Geometry: final body of the model. Coordinates: model frame, mm. Give positions to 0.01 mm unless a question says otherwise; leave off trailing zeros. Loops run counter-clockwise (first coordinate to the right, second up) from the corner with the lowest first, then second, coordinate; pieces in that order, holes last. Notation, with made-up numbers: (44.25, 73) - (49.25, 73) arc R17 ccw to (49.25, 83) - close; hole circle Ø11 at (83.5, 42.5). An arc over 180 degrees is marked (long way). Answer in a Markdown table with one row per item.
from build123d import *

# Parameters (mm, degrees)
F0_W           = 48
F0_H           = 48
F1_DEPTH       = 48
F2_R           = 1
F3_R           = 1
F4_T1_DEPTH    = 46
F4_T3_DEPTH    = 46
F4_T5_DEPTH    = 46
F4_S9_W        = 1
F4_S9_H        = 1
F4_T10_DEPTH   = 1
F4_S15_W       = 1
F4_S15_H       = 1
F4_T16_DEPTH   = 1
F4_S21_W       = 1
F4_S21_H       = 1
F4_T22_DEPTH   = 1
F4_S27_W       = 1
F4_S27_H       = 1
F4_T28_DEPTH   = 1
F4_T32_ANGLE   = 90
F4_T34_ANGLE   = 90
F6_D           = 18
F6_CSINK_D     = 36
F6_CSINK_ANGLE = 45


# Not quite as in the source:
# - a fillet or chamfer that OpenCascade refuses, or shapes differently, is made with other operations: its cross-section is extruded or revolved along the edge and cut away or added


with BuildPart() as f1:
    # F0 (on Front) → F1 (new body)
    with BuildSketch(Plane.XZ):
        Rectangle(F0_W, F0_H)
    extrude(amount=F1_DEPTH)

    # F2
    f2_edges = [f1.edges().sort_by_distance(p)[0] for p in [
        (24, -24, 24),
    ]]
    fillet(f2_edges, radius=F2_R)

    # F3
    f3_edges = [f1.edges().sort_by_distance(p)[0] for p in [
        (-24, -24, 24),
        (-0.5, 0, 24),
        (-0.5, -48, 24),
    ]]
    fillet(f3_edges, radius=F3_R)

    # F4: fillet of radius 1 on 8 edges, made by hand

    # F4_s2 → F4_t1 (cut)
    with BuildSketch(Plane.XY.offset(-23)):
        with BuildLine():
            ThreePointArc((-23, -48), (-23.7071067812, -47.7071067812), (-24, -47))
            Line((-24, -47), (-24, -48))
            Line((-24, -48), (-23, -48))
        make_face()
        with BuildLine():
            ThreePointArc((-23, 0), (-23.7071067812, -0.2928932188), (-24, -1))
            Line((-24, -1), (-24, 0))
            Line((-24, 0), (-23, 0))
        make_face()
    extrude(amount=F4_T1_DEPTH, mode=Mode.SUBTRACT)

    # F4_s4 → F4_t3 (cut)
    with BuildSketch(Plane.YZ.offset(-23)):
        with BuildLine():
            ThreePointArc((0, -23), (-0.2928932188, -23.7071067812), (-1, -24))
            Line((-1, -24), (0, -24))
            Line((0, -24), (0, -23))
        make_face()
        with BuildLine():
            ThreePointArc((-48, -23), (-47.7071067812, -23.7071067812), (-47, -24))
            Line((-47, -24), (-48, -24))
            Line((-48, -24), (-48, -23))
        make_face()
    extrude(amount=F4_T3_DEPTH, mode=Mode.SUBTRACT)

    # F4_s6 → F4_t5 (cut)
    with BuildSketch(Plane.XZ.offset(1)):
        with BuildLine():
            ThreePointArc((-24, -23), (-23.7071067812, -23.7071067812), (-23, -24))
            Line((-23, -24), (-24, -24))
            Line((-24, -24), (-24, -23))
        make_face()
        with BuildLine():
            ThreePointArc((24, -23), (23.7071067812, -23.7071067812), (23, -24))
            Line((23, -24), (24, -24))
            Line((24, -24), (24, -23))
        make_face()
    extrude(amount=F4_T5_DEPTH, mode=Mode.SUBTRACT)


with BuildPart() as f4_tool8:
    # F4_s9 → F4_t10 (new body)
    with BuildSketch(Plane.XZ.offset(1)):
        with Locations((-23.5, 23.5)):
            Rectangle(F4_S9_W, F4_S9_H)
    extrude(amount=-F4_T10_DEPTH)

    # F4_s11 → F4_t12 (revolve, cut)
    with BuildSketch(Plane(origin=(-23, -1, 23), x_dir=(0.7071067812, 0, -0.7071067812), z_dir=(0.7071067812, 0, 0.7071067812))):
        with BuildLine():
            ThreePointArc((0, -1), (1, 0), (0, 1))
            Line((0, 1), (0, -1))
        make_face()
    revolve(axis=Axis((-23, -1, 23), (0, 1, 0)), mode=Mode.SUBTRACT)


with BuildPart() as f1_1:
    add(f1.part)

    # F4_t7: cut F4_tool8
    add(f4_tool8.part, mode=Mode.SUBTRACT)


with BuildPart() as f4_tool14:
    # F4_s15 → F4_t16 (new body)
    with BuildSketch(Plane.XZ.offset(47)):
        with Locations((-23.5, 23.5)):
            Rectangle(F4_S15_W, F4_S15_H)
    extrude(amount=F4_T16_DEPTH)

    # F4_s17 → F4_t18 (revolve, cut)
    with BuildSketch(Plane(origin=(-23, -47, 23), x_dir=(0.7071067812, 0, -0.7071067812), z_dir=(-0.7071067812, 0, -0.7071067812))):
        with BuildLine():
            ThreePointArc((0, -1), (1, 0), (0, 1))
            Line((0, 1), (0, -1))
        make_face()
    revolve(axis=Axis((-23, -47, 23), (0, -1, 0)), mode=Mode.SUBTRACT)


with BuildPart() as f1_2:
    add(f1_1.part)

    # F4_t13: cut F4_tool14
    add(f4_tool14.part, mode=Mode.SUBTRACT)


with BuildPart() as f4_tool20:
    # F4_s21 → F4_t22 (new body)
    with BuildSketch(Plane.XZ.offset(47)):
        with Locations((-23.5, -23.5)):
            Rectangle(F4_S21_W, F4_S21_H)
    extrude(amount=F4_T22_DEPTH)

    # F4_s23 → F4_t24 (revolve, cut)
    with BuildSketch(Plane(origin=(-23, -47, -23), x_dir=(0.7071067812, 0, 0.7071067812), z_dir=(0.7071067812, 0, -0.7071067812))):
        with BuildLine():
            ThreePointArc((0, -1), (1, 0), (0, 1))
            Line((0, 1), (0, -1))
        make_face()
    revolve(axis=Axis((-23, -47, -23), (0, -1, 0)), mode=Mode.SUBTRACT)


with BuildPart() as f1_3:
    add(f1_2.part)

    # F4_t19: cut F4_tool20
    add(f4_tool20.part, mode=Mode.SUBTRACT)


with BuildPart() as f4_tool26:
    # F4_s27 → F4_t28 (new body)
    with BuildSketch(Plane.XZ.offset(1)):
        with Locations((-23.5, -23.5)):
            Rectangle(F4_S27_W, F4_S27_H)
    extrude(amount=-F4_T28_DEPTH)

    # F4_s29 → F4_t30 (revolve, cut)
    with BuildSketch(Plane(origin=(-23, -1, -23), x_dir=(0.7071067812, 0, 0.7071067812), z_dir=(-0.7071067812, 0, 0.7071067812))):
        with BuildLine():
            ThreePointArc((0, -1), (1, 0), (0, 1))
            Line((0, 1), (0, -1))
        make_face()
    revolve(axis=Axis((-23, -1, -23), (0, 1, 0)), mode=Mode.SUBTRACT)


with BuildPart() as f1_4:
    add(f1_3.part)

    # F4_t25: cut F4_tool26
    add(f4_tool26.part, mode=Mode.SUBTRACT)

    # F4_s31 → F4_t32 (revolve, cut)
    with BuildSketch(Plane.XZ.offset(1)):
        with BuildLine():
            ThreePointArc((24, -23), (23.7071067812, -23.7071067812), (23, -24))
            Line((23, -24), (24, -24))
            Line((24, -24), (24, -23))
        make_face()
    revolve(axis=Axis((23, -1, -24), (0, 0, 1)), revolution_arc=F4_T32_ANGLE, mode=Mode.SUBTRACT)

    # F4_s33 → F4_t34 (revolve, cut)
    with BuildSketch(Plane.XZ.offset(47)):
        with BuildLine():
            ThreePointArc((24, -23), (23.7071067812, -23.7071067812), (23, -24))
            Line((23, -24), (24, -24))
            Line((24, -24), (24, -23))
        make_face()
    revolve(axis=Axis((23, -47, -24), (0, 0, -1)), revolution_arc=F4_T34_ANGLE, mode=Mode.SUBTRACT)

    # F6 (through all)
    with Locations(Plane.XY.offset(24)):
        with Locations((0, -24)):
            CounterSinkHole(F6_D / 2, F6_CSINK_D / 2, counter_sink_angle=F6_CSINK_ANGLE)


solid = f1_4.part
Q1. Cut plane C-C (x = 0). Output: boundary loops of the cut face in (y, z).
Check values:
| item | result |
|---|---|
| outline | (-48, -23) arc R1 ccw to (-47, -24) - (-33, -24) - (-33, 2.27) - (-42, 24) - (-47, 24) arc R1 ccw to (-48, 23) - close; (-15, -24) - (-1, -24) arc R1 ccw to (0, -23) - (0, 23) arc R1 ccw to (-1, 24) - (-6, 24) - (-15, 2.27) - close |
Q2. Cut plane D-D (z = 10). Output: boundary loops of the cut face in (x, y).
Check values:
| item | result |
|---|---|
| outline | (-24, -47) arc R1 ccw to (-23, -48) - (23, -48) arc R1 ccw to (24, -47) - (24, -1) arc R1 ccw to (23, 0) - (-23, 0) arc R1 ccw to (-24, -1) - close; hole circle Ø24.4 at (0, -24) |
Q3. Draft query along X for faces 1 (the cylindrical face through (1.172, -15.077, -11.048)), 2 (the conical face through (-6.148, -14.356, 8.156)), 3 (the flat face through (24, -24, 0)), 4 (the flat face through (-16, -13, 24)). Return one class per face: pulls with the +X half, pulls with the -X half, needs draft (parallel to the pull), parting line crosses it, or undercut.
Check values:
| item | result |
|---|---|
| face 1 | undercut |
| face 2 | undercut |
| face 3 | pulls with the +X half |
| face 4 | needs draft |
Q4. Material intervals for line 1 along X through (y, z) = (-24, -15.75); line 2 along Y through (x, z) = (0, -4.5); line 3 along X through (y, z) = (-16, 3.5), sorted ascending.
Check values:
| item | result |
|---|---|
| line 1 | -24 to -9, 9 to 24 |
| line 2 | -48 to -33, -15 to 0 |
| line 3 | -24 to -5.14, 5.14 to 24 |
Q5. First-contact query: pin 1 (16 mm diameter, centred on x = 0, y = -24, fed in from -Z); pin 2 (1.5 mm diameter, centred on x = -2, y = -37, fed in from +Z). Flat tips, straight axial feed; report the tip coordinate or a pass-through.
Check values:
| item | result |
|---|---|
| pin 1 | through |
| pin 2 | z = 14.11 |
Q6. Cut plane A-A (z = 1). Output: boundary loops of the cut face in (x, y), and give its area (3 significant figures).
Check values:
| item | result |
|---|---|
| outline | (-24, -47) arc R1 ccw to (-23, -48) - (23, -48) arc R1 ccw to (24, -47) - (24, -1) arc R1 ccw to (23, 0) - (-23, 0) arc R1 ccw to (-24, -1) - close; hole circle Ø18 at (0, -24) |
| area | 2,050 mm² |
Q7. Cut plane B-B (y = -24). Output: boundary loops of the cut face in (x, z).
Check values:
| item | result |
|---|---|
| outline | (-24, -23) arc R1 ccw to (-23, -24) - (-9, -24) - (-9, 2.27) - (-18, 24) - (-23, 24) arc R1 ccw to (-24, 23) - close; (9, -24) - (23, -24) arc R1 ccw to (24, -23) - (24, 23) arc R1 ccw to (23, 24) - (18, 24) - (9, 2.27) - close |
